Autodesk Inventor part; units mm, degrees
ref_plane "WorkPlane1" through (0, 0, 0) normal (0, 0, 1) x (1, 0, 0)
ref_plane "MSC_PF1" through (0, 0, 0) normal (1, 0, 0) x (0, 1, 0)
ref_plane "MSC_PT1" through (0, 0, 0) normal (0, 0, -1) x (-1, 0, 0)
ref_plane "WorkPlane1" through (0, 0, 0) normal (0, 0, 1) x (1, 0, 0)
sketch "Sketch1" plane through (0, 0, 0) normal (0, 0, 1) x (1, 0, 0)
  point P0 (0, 0)
sketch "Sketch2" plane through (0, 0, 0) normal (0, 0, 1) x (1, 0, 0)
  line L0 (-8, 4.6189) -> (-8, -4.6189)
  line L1 (0, 9.2375) -> (-8, 4.6189)
  line L2 (8, 4.6189) -> (0, 9.2375)
  line L3 (8, -4.6189) -> (8, 4.6189)
  line L4 (0, -9.2375) -> (8, -4.6189)
  line L5 (-8, -4.6189) -> (0, -9.2375)
  circle A0 centre (0, 0) radius 8 construction
  dimension "d1" = 16
  dimension "d29" = 0
  dimension "d30" = 0
extrude "Extrusion1" add sketch "Sketch2" along normal blind 6.4
sketch "Sketch3" plane through (0, 0, 0) normal (1, 0, 0) x (0, 1, 0)
  line L0 (8, 6.4) -> (9.3375, 6.4)
  line L1 (9.3375, 5.6278) -> (8, 6.4)
  line L2 (9.3375, 6.4) -> (9.3375, 5.6278)
  line L3 (0, -1.28) -> (0, 7.68)
  line L4 (9.2375, 0) -> (9.2375, 6.4)
  dimension "d25" = 0.1
  dimension "d26" = 0
  dimension "d27" = 60
  dimension "d28" = 8
revolve "Revolution1" cut sketch "Sketch3" angle 360 about axis through (0, 0, -10) along (0, 0, 1)
sketch "Sketch4" plane through (0, 0, 0) normal (1, 0, 0) x (0, 1, 0)
  line L0 (0, -100) -> (0, 0)
  line L1 (-5, -100) -> (0, -100)
  line L2 (-5, 0) -> (-5, -100)
  line L3 (0, 0) -> (-5, 0)
  line L4 (0, -100) -> (0, 0)
  line L5 (-6, 0) -> (1, 0)
  line L6 (0, -120) -> (0, 20)
  dimension "d18" = 5
  dimension "d20" = 100
  dimension "d33" = 0
  dimension "d34" = 0
revolve "Revolution2" add sketch "Sketch4" angle 360 about axis through (0, 0, -100) along (0, 0, -1)
chamfer "Chamfer1" distance 0.75 angle 45 1 edges at (0, 5, -100)
fillet "Fillet1" radius 0.4 1 edges at (0, 5, 0)
thread "Thread1"
ref_plane "MSC_PF1" through (0, 0, 0) normal (1, 0, 0) x (0, 1, 0)
ref_plane "MSC_PT1" through (0, 0, 0) normal (0, 0, -1) x (-1, 0, 0)
equation "\"d22\" = 0.5 * PTC"
equation "\"d23\" = 0.5 * PTC"
equation "\"d24\" = r"
equation "\"d1\" = ParS"
equation "\"d6\" = ParK"
equation "\"b\" = NLG - 2 * PTC"
equation "\"d28\" = 0.5 * ParS"
equation "\"d18\" = 0.5 * NND"
equation "\"d20\" = NLG"
equation "\"NLG\" = 100"
equation "\"PTC\" = 1.5"
equation "\"ParK\" = 6.4"
equation "\"ParS\" = 16"
equation "\"msp_es\" = 0.577367 * ParS"
equation "\"r\" = 0.4"
equation "\"K1\" = 4.17"
properties part number "DIN EN ISO 4018 - M10x100" material "Stainless Steel"
For this review, take the finished solid that the model builds, in its own axes (mm). A direction names the side the tool comes from. Round coordinates to 2 decimals unless told otherwise and drop trailing zeros. Loops run counter-clockwise (first coordinate to the right, second up) from the corner with the lowest first, then second, coordinate; pieces in that order, holes last. Notation, with made-up numbers: (46.5, 1.5) - (62.5, 1.5) arc R15 ccw to (62.5, 27.5) - close; hole circle Ø5 at (71.5, 51). An arc over 180 degrees is marked (long way). Put each result on its own line as item: value. Start each with the question number.
1. For probe 1 along Z at (x, y) = (-2.25, -7.25); probe 2 along Y at (x, z) = (-3, -87.5), list the stretches that pass through material, from the lowest coordinate up. Write a range as [from, to].
2. Insertion check: P1, Ø8, axis at x = 6, z = -7, coming from the +Y side; P2, Ø5, axis at y = -5.5, z = -15.5, coming from the -X side; P3, Ø8, axis at x = 3.5, y = 3.5, coming from the -Z side; P4, Ø2, axis at x = 2.5, y = -7, coming from the -Z side. Each pin has a flat end and moves straight along its axis. Give the tip position at first contact, or say it passes through.
3. For faces 1 (the flat face through (-4, -4, 0)), 2 (the conical face through (7.179, 4.168, 6.226)), list the 3-axis set-ups (+Z, -Z, +X, -X, +Y, -Y) from which the entire face can be reached by the end or side of a thin tool; tool diameter is ignored.
4. Consider section A-A on z = -67.5. State the section outline as (x, y) points.
Result sheet:
1. probe 1: [0, 6.4]
1. probe 2: [-4, 4]
2. P1: y = 4.58
2. P2: x = -4
2. P3: z = -100
2. P4: z = 0
3. face 1: -Z
3. face 2: +Z, +X, +Y
4. outline: circle Ø10 at (0, 0)
